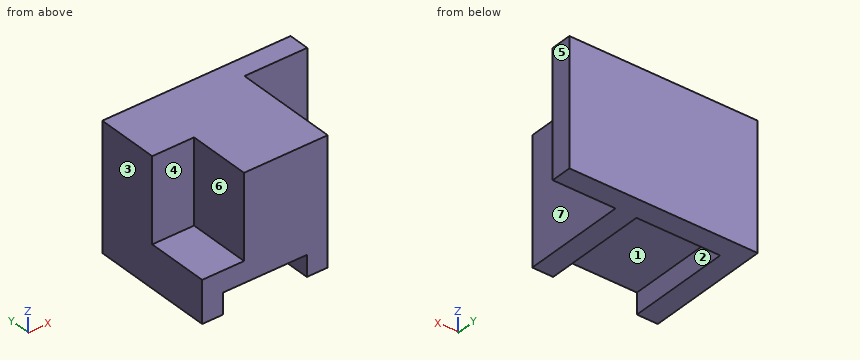
from build123d import *

# Parameters (mm, degrees)
F1_DEPTH = 60
F0_W     = 20
F0_H     = 40
F0_W_2   = 30
F0_H_2   = 60
F0_W_3   = 40
F0_H_3   = 10
F2_DEPTH = 10
F3_DEPTH = 30


with BuildPart() as f1:
    # F0 (on Front) → F1 (new body)
    with BuildSketch(Plane.XZ):
        Polygon((14.700101, 32.967453), (-25.299899, 32.967453), (-25.299899, -7.032547), (-45.299899, -7.032547), (-45.299899, -27.032547), (-35.299899, -27.032547), (-35.299899, -17.032547), (4.700101, -17.032547), (4.700101, -27.032547), (14.700101, -27.032547), align=None)
    extrude(amount=F1_DEPTH)

    # F0 (on Front) → F2 (join)
    with BuildSketch(Plane.XZ):
        with Locations((-35.299899, 12.967453)):
            Rectangle(F0_W, F0_H)
        Polygon((14.700101, 32.967453), (-25.299899, 32.967453), (-25.299899, -7.032547), (-45.299899, -7.032547), (-45.299899, -27.032547), (-35.299899, -27.032547), (-35.299899, -17.032547), (4.700101, -17.032547), (4.700101, -27.032547), (14.700101, -27.032547), align=None)
        with Locations((29.700101, 2.967453)):
            Rectangle(F0_W_2, F0_H_2)
        with Locations((-15.299899, -22.032547)):
            Rectangle(F0_W_3, F0_H_3)
    extrude(amount=F2_DEPTH)

    # F0 (on Front) → F3 (join)
    with BuildSketch(Plane.XZ):
        with Locations((-35.299899, 12.967453)):
            Rectangle(F0_W, F0_H)
    extrude(amount=F3_DEPTH)


solid = f1.part
Design review of the part built by this model. Coordinates are the model's own, in mm. Face numbers are marked on the shaded views. A direction names the side the tool comes from. Coordinates: 2 decimals unless noted, no trailing zeros. Order: outer loops, then holes, each group sorted by start corner. A loop starts at its lowest first (then second) coordinate and runs counter-clockwise, first axis right, second up. Notation, with made-up numbers: (66, -25.75) -> (75, -25.75) arc R7 ccw to (75, -16.75) -> close; hole circle Ø5 at (23, 63). An arc over 180 degrees is marked (long way). One line per item, written item: value.
1) Machinability: for the marked faces 5, 6 and 7, which of the approach directions +Z, -Z, +X, -X, +Y, -Y give a long, thin tool a straight path to every point of the face, cutting with its end or side? Answer none if there is none.
Output values:
face 5: +Z, -Z, +X, +Y, -Y
face 6: +Z, -X, -Y
face 7: +Z, -Z, +X, -Y
2) To check wall thickness, follow probe 1 along Z at (x, y) = (-23, -34.5); probe 2 along Y at (x, z) = (-30.5, 4.5); probe 3 along X at (y, z) = (-24.5, -21). State the ranges of each line that lie inside material, in increasing order. Write a range as [from, to].
Output values:
probe 1: z = [-17.03, 32.97]
probe 2: y = [-30, 0]
probe 3: x = [-45.3, -35.3], [4.7, 14.7]
3) We need section D-D, the plane z = -22. Give the boundary of the cut face in (x, y).
Output values:
outline: (-45.3, -60) -> (-35.3, -60) -> (-35.3, -10) -> (4.7, -10) -> (4.7, -60) -> (14.7, -60) -> (14.7, -10) -> (44.7, -10) -> (44.7, 0) -> (-45.3, 0) -> close
4) Draft analysis for pull direction X (two halves, no side actions). For the marked faces 1, 2, 3 and 4, state which applies: +X half, -X half, draft (parallel to the pull), parting line (faces both ways), or undercut.
Output values:
face 1: undercut
face 2: undercut
face 3: -X half
face 4: draft
5) We need section B-B, the plane z = -1. Give the boundary of the cut face in (x, y), then the cut area to 3 significant figures.
Output values:
outline: (-45.3, -30) -> (-25.3, -30) -> (-25.3, -60) -> (14.7, -60) -> (14.7, -10) -> (44.7, -10) -> (44.7, 0) -> (-45.3, 0) -> close
area: 3,300 mm2
6) Clearance check with flat-ended pins moving along their axes: P1, Ø15, axis at y = -32.5, z = -9.5, coming from the +X side; P2, Ø6, axis at x = -31.5, z = 5.5, coming from the -Y side; P3, Ø2, axis at y = -32.5, z = -3.5, coming from the -X side. State where each tip first meets the part, or that it passes through.
Output values:
P1: stops at x = 14.7
P2: stops at y = -30
P3: stops at x = -25.3
7) We need section A-A, the plane y = -53. Give the boundary of the cut face in (x, z), then the cut area to 3 significant figures.
Output values:
outline: (-45.3, -27.03) -> (-35.3, -27.03) -> (-35.3, -17.03) -> (4.7, -17.03) -> (4.7, -27.03) -> (14.7, -27.03) -> (14.7, 32.97) -> (-25.3, 32.97) -> (-25.3, -7.03) -> (-45.3, -7.03) -> close
area: 2,400 mm2
8) We need section C-C, the plane x = 28.5. Give the boundary of the cut face in (y, z).
Output values:
outline: (-10, -27.03) -> (0, -27.03) -> (0, 32.97) -> (-10, 32.97) -> close
